Could you check a few things on this model? Use its own coordinates, in mm. Face numbers are marked on the shaded views. A direction names the side the tool comes from. Coordinates: 2 decimals unless noted, no trailing zeros. Write each loop counter-clockwise with the first axis right and the second up, starting at its lowest first coordinate (ties: lowest second). Pieces come first, ordered by that corner, then holes.
Item 1: If I drill on probe 1 along Z at (x, y) = (4.35, -36.9); probe 2 along Y at (x, z) = (3.25, -0.9); probe 3 along X at (y, z) = (-37.5, -35.5), over which ranges is the centre line in solid material (lowest first)?
Item 2: For P1, Ø2, axis at x = -3.25, y = 0, coming from the +Z side; P2, Ø4, axis at x = -1.5, y = -27.5, coming from the -Z side; P3, Ø4.5, axis at x = -2.5, y = -23, coming from the -Z side; P4, Ø6.5, axis at x = -8, z = -2.5, coming from the +Y side, each with a flat end and sliding along its axis, tell me the tip position at first contact or that it passes through.
Item 3: Thinking about a two-plate mould opening in Z: for the marked faces 4, 5 and 6, which applies, +Z half, -Z half, draft (parallel to the pull), parting line (faces both ways), or undercut?
Item 4: I want a section at D-D on z = -37.5. Please give me the cut outline in (x, y).
Item 5: I want a section at B-B on y = 0. Please give me the cut outline in (x, z).
Item 6: I want a section at A-A on x = -3.25. Please give me the cut outline in (y, z).
Item 7: Which directions (+Z, -Z, +X, -X, +Y, -Y) give clear straight access to the entire face, cutting with the end or side of a thin tool? Please do the marked faces 1, 2 and 3.
Item 8: I want a section at C-C on z = -7.5. Please give me the cut outline in (x, y), then the cut area to 3 significant figures.
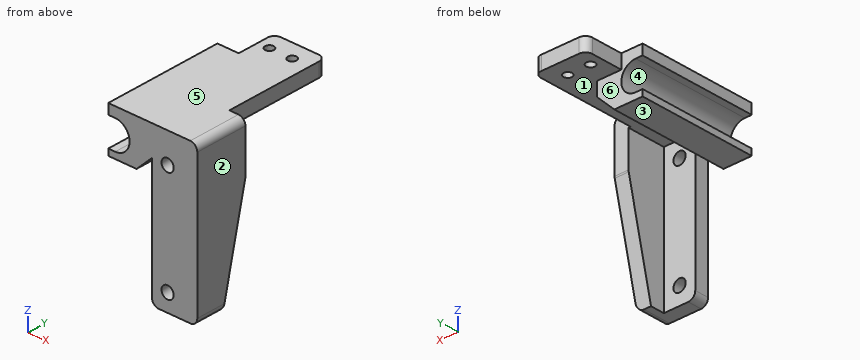
from build123d import *

# Parameters (mm, degrees)
SKETCH1_W           = 14.8
SKETCH1_H           = 45
SKETCH1_R           = 1.25
BOSS_EXTRUDE1_DEPTH = 2
BOSS_EXTRUDE2_DEPTH = 34
CHAMFER2_SIZE       = 5
SKETCH3_W           = 9
SKETCH3_H           = 44.5
SKETCH3_R           = 1.75
BOSS_EXTRUDE3_DEPTH = 4
BOSS_EXTRUDE4_DEPTH = 15
CHAMFER3_SIZE       = 7
CHAMFER3_SIZE2      = 30
FILLET3_R           = 2
FILLET4_R           = 2


with BuildPart() as part:
    # Sketch1 → Boss-Extrude1 (new body, symmetric)
    with BuildSketch(Plane.XY):
        with Locations((0.85, -17.5)):
            Rectangle(SKETCH1_W, SKETCH1_H)
        with Locations((-3.25, 0)):
            Circle(SKETCH1_R, mode=Mode.SUBTRACT)
        with Locations((3.25, 0)):
            Circle(SKETCH1_R, mode=Mode.SUBTRACT)
    extrude(amount=BOSS_EXTRUDE1_DEPTH, both=True)

    # Sketch2 → Boss-Extrude2 (add)
    with BuildSketch(Plane.XZ.offset(40)):
        with BuildLine():
            Line((-6.55, -2), (-6.55, 2))
            Line((-6.55, 2), (-12.65, 2))
            Line((-12.65, 2), (-12.65, -0.9))
            Line((-12.65, -0.9), (-10.65, -0.9))
            ThreePointArc((-10.65, -0.9), (-6.55, -5), (-10.65, -9.1))
            Line((-10.65, -9.1), (-12.65, -9.1))
            Line((-12.65, -9.1), (-12.65, -10.9))
            Line((-12.65, -10.9), (0.45, -10.9))
            Line((0.45, -10.9), (0.45, -2))
            Line((0.45, -2), (-6.55, -2))
        make_face()
    extrude(amount=-BOSS_EXTRUDE2_DEPTH)

    # Chamfer2
    chamfer2_edges = [part.edges().sort_by_distance(p)[0] for p in [
        (0.45, -23, -10.9),
    ]]
    chamfer(chamfer2_edges, length=CHAMFER2_SIZE)

    # Sketch3 → Boss-Extrude3 (add)
    with BuildSketch(Plane.XZ.offset(40)):
        with Locations((4.35, -20.25)):
            Rectangle(SKETCH3_W, SKETCH3_H)
        with Locations((4.35, -37.5)):
            Circle(SKETCH3_R, mode=Mode.SUBTRACT)
        with Locations((4.35, -6.5)):
            Circle(SKETCH3_R, mode=Mode.SUBTRACT)
    extrude(amount=-BOSS_EXTRUDE3_DEPTH)

    # Sketch4 → Boss-Extrude4 (add)
    with BuildSketch(Plane(origin=(0, -40, 0), x_dir=(-1, 0, 0), z_dir=(0, 1, 0))):
        Polygon((-8.85, -42.5), (-12.85, -42.5), (-12.85, 2), (-8.85, 2), (-8.25, 2), (-8.25, -2), (-8.85, -2), align=None)
    extrude(amount=BOSS_EXTRUDE4_DEPTH)

    # Chamfer3
    chamfer3_edges = [part.edges().sort_by_distance(p)[0] for p in [
        (10.85, -25, -42.5),
    ]]
    chamfer3_side = [part.faces().sort_by_distance(p)[0] for p in [
        (0.048494332, -38, -42.5),
    ]]
    chamfer(chamfer3_edges, length=CHAMFER3_SIZE, length2=CHAMFER3_SIZE2, reference=chamfer3_side[0])

    # Fillet3
    fillet3_edges = [part.edges().sort_by_distance(p)[0] for p in [
        (10.85, -25, -12.5),
        (12.85, -36, -42.5),
        (-0.15, -38, -42.5),
        (12.85, -32.5, 2),
    ]]
    fillet(fillet3_edges, radius=FILLET3_R)

    # Fillet4
    fillet4_edges = [part.edges().sort_by_distance(p)[0] for p in [
        (-6.55, 5, 0),
        (8.25, 5, 0),
    ]]
    fillet(fillet4_edges, radius=FILLET4_R)


solid = part.part
Response values:
1. probe 1: z = -42.5 to -39.25, -35.75 to -8.25, -4.75 to 2
1. probe 2: y = -40 to -1.25, 1.25 to 5
1. probe 3: x = -0.15 to 12.85
2. P1: passes through
2. P2: stops at z = -9.85
2. P3: stops at z = -10.9
2. P4: stops at y = 4.99
3. face 4: undercut
3. face 5: +Z half
3. face 6: draft
4. outline: (-0.15, -40) - (2.6, -40) - (2.6, -36) - (-0.15, -36) - close; (6.1, -40) - (12.85, -40) - (12.85, -30.83) - (8.85, -30.83) - (8.85, -36) - (6.1, -36) - close
5. outline: (-6.55, -2) - (-4.5, -2) - (-4.5, 2) - (-6.55, 2) - close; (-2, -2) - (2, -2) - (2, 2) - (-2, 2) - close; (4.5, -2) - (8.25, -2) - (8.25, 2) - (4.5, 2) - close
6. outline: (-40, -9.6) - (-6, -9.6) - (-6, -2) - (-1.25, -2) - (-1.25, 2) - (-40, 2) - close; (1.25, -2) - (5, -2) - (5, 2) - (1.25, 2) - close
7. face 1: -Z, +Y
7. face 2: +Z, -Z, +X, +Y, -Y
7. face 3: -Z, -X, +Y, -Y
8. outline: (-7.4, -40) - (-1.15, -40) - (-1.15, -6) - (-7.4, -6) - close; (-0.15, -40) - (2.91, -40) - (2.91, -36) - (-0.15, -36) - close; (5.79, -40) - (12.85, -40) - (12.85, -25) - (8.85, -25) - (8.85, -36) - (5.79, -36) - close
8. area: 297 mm2
